Can you work these out from the model? Positions are in its coordinate system, mm. Coordinates: 2 decimals unless noted, no trailing zeros. Answer in a Markdown table with one row per item. Add a question column.
1. Will these pins go through, and if not, where does the flat tip stop? pin 1 (1.6 mm diameter, centred on y = 1, z = -103.5, fed in from -X); pin 2 (1 mm diameter, centred on x = -102.5, y = 2.5, fed in from -Z); pin 3 (1 mm diameter, centred on y = 1.5, z = 103.5, fed in from +X).
2. If I drill on line 1 along Z through (x, y) = (94, 0.1), over which ranges is the centre line in solid material (lowest first)? Write a range as [from, to].
3. We'd pull the mould along X, two halves only. Please class faces 1 (the face through (-94.548, 1.61, -91.343)), 2 (the face through (96.31, 1.57, -96.12)), 3 (the face through (-1, 0, -1)): pulls with the +X half, pulls with the -X half, needs draft (parallel to the pull), parting line crosses it, or undercut.
from build123d import *

# Parameters (mm, degrees)
BOSS_EXTRUDE1_DEPTH = 3.175
CUT_EXTRUDE1_REACH  = 5.175
SKETCH3_R           = 2.286


with BuildPart() as part:
    # Sketch1 → Boss-Extrude1 (new body)
    with BuildSketch(Plane(origin=(0, 0, 0), x_dir=(1, 0, 0), z_dir=(0, 1, 0))):
        Polygon((-91.233267746, 104.4575), (-91.233267746, 101.1555), (-101.1555, 91.321365209), (-104.4575, 91.321365209), (-104.4575, -91.233267746), (-101.1555, -91.233267746), (-91.321365209, -101.1555), (-91.321365209, -104.4575), (91.233267746, -104.4575), (91.233267746, -101.1555), (101.1555, -91.321365209), (104.4575, -91.321365209), (104.4575, 91.233267746), (101.1555, 91.233267746), (91.321365209, 101.1555), (91.321365209, 104.4575), align=None)
    extrude(amount=BOSS_EXTRUDE1_DEPTH)

    # Sketch3 → Cut-Extrude1 (cut, up to next)
    with BuildSketch(Plane(origin=(0, 3.175, 0), x_dir=(1, 0, 0), z_dir=(0, 1, 0)), mode=Mode.PRIVATE) as cut_extrude1_sk1:
        with Locations((-92.73413, 92.73413)):
            Circle(SKETCH3_R)
    cut_extrude1_tool1 = extrude(cut_extrude1_sk1.sketch, amount=-CUT_EXTRUDE1_REACH, mode=Mode.PRIVATE) & part.part
    add(cut_extrude1_tool1.solids().sort_by_distance((-92.73413, 3.175, -92.73413))[0], mode=Mode.SUBTRACT)
    # Sketch3 → Cut-Extrude1 (cut, up to next)
    with BuildSketch(Plane(origin=(0, 3.175, 0), x_dir=(1, 0, 0), z_dir=(0, 1, 0)), mode=Mode.PRIVATE) as cut_extrude1_sk2:
        with Locations((92.73413, 92.73413)):
            Circle(SKETCH3_R)
    cut_extrude1_tool2 = extrude(cut_extrude1_sk2.sketch, amount=-CUT_EXTRUDE1_REACH, mode=Mode.PRIVATE) & part.part
    add(cut_extrude1_tool2.solids().sort_by_distance((92.73413, 3.175, -92.73413))[0], mode=Mode.SUBTRACT)
    # Sketch3 → Cut-Extrude1 (cut, up to next)
    with BuildSketch(Plane(origin=(0, 3.175, 0), x_dir=(1, 0, 0), z_dir=(0, 1, 0)), mode=Mode.PRIVATE) as cut_extrude1_sk3:
        with Locations((92.73413, -92.73413)):
            Circle(SKETCH3_R)
    cut_extrude1_tool3 = extrude(cut_extrude1_sk3.sketch, amount=-CUT_EXTRUDE1_REACH, mode=Mode.PRIVATE) & part.part
    add(cut_extrude1_tool3.solids().sort_by_distance((92.73413, 3.175, 92.73413))[0], mode=Mode.SUBTRACT)
    # Sketch3 → Cut-Extrude1 (cut, up to next)
    with BuildSketch(Plane(origin=(0, 3.175, 0), x_dir=(1, 0, 0), z_dir=(0, 1, 0)), mode=Mode.PRIVATE) as cut_extrude1_sk4:
        with Locations((-92.73413, -92.73413)):
            Circle(SKETCH3_R)
    cut_extrude1_tool4 = extrude(cut_extrude1_sk4.sketch, amount=-CUT_EXTRUDE1_REACH, mode=Mode.PRIVATE) & part.part
    add(cut_extrude1_tool4.solids().sort_by_distance((-92.73413, 3.175, 92.73413))[0], mode=Mode.SUBTRACT)


solid = part.part
Answers follow:
| question | item | result |
|---|---|---|
| 1 | pin 1 | stops at x = -91.23 |
| 1 | pin 2 | stops at z = -91.32 |
| 1 | pin 3 | stops at x = 91.23 |
| 2 | line 1 | z = [-98.45, -94.64], [-90.83, 90.83], [94.64, 98.41] |
| 3 | face 1 | undercut |
| 3 | face 2 | pulls with the +X half |
| 3 | face 3 | needs draft |
